from build123d import *

# Parameters (mm, degrees)
BOX_W              = 13.4
BOX_H              = 13.4
BOX_DEPTH          = 14
SKETCH001_R        = 20
POCKET_DEPTH       = 6
POLARPATTERN_COUNT = 5


with BuildPart() as cube:
    # Box → Box (new body)
    with BuildSketch(Plane(origin=(-6.7, -6.7, 10), x_dir=(1, 0, 0), z_dir=(0, 0, 1))):
        with Locations((6.7, 6.7)):
            Rectangle(BOX_W, BOX_H)
    extrude(amount=BOX_DEPTH)


with BuildPart() as body:
    # Sketch → Revolve (revolve)
    with BuildSketch(Plane.XZ):
        with BuildLine():
            Line((78.70723, 18.37), (90, 18.37))
            Line((90, 18.37), (82.032315, 21.27))
            Line((82.032315, 21.27), (82.032315, 23.77))
            Line((82.032315, 23.77), (90, 26.67))
            Line((90, 26.67), (4.86, 26.67))
            Line((4.86, 26.67), (4.86, 10.010664))
            Line((4.86, 10.010664), (11.05, 10.010664))
            Line((11.05, 10.010664), (11.05, 18.37))
            add(Edge.make_bspline(
                [(78.70723, 18.37), (58.452015, 25.146616), (31.574902, 25.049244), (11.05, 18.37)],
                knots=[0, 0, 0, 0, 1, 1, 1, 1], degree=3))
        make_face()
    revolve(axis=Axis((0, 0, 0), (0, 0, 1)))

    # Cut: cut Cube
    add(cube.part, mode=Mode.SUBTRACT)

    # Sketch001 (on Face12 of BaseFeature) → Pocket (cut)
    with BuildSketch(Plane.XY.offset(26.67)):
        with Locations((-32.618477, 27.97224)):
            Circle(SKETCH001_R)
    pocket = extrude(amount=-POCKET_DEPTH, mode=Mode.SUBTRACT)

    # PolarPattern: Pocket ×5 about axis
    polarpattern_axis = Axis((0, 0, 26.67), (0, 0, 1))
    for i in range(1, POLARPATTERN_COUNT):
        add(pocket.rotate(polarpattern_axis, i * 360 / POLARPATTERN_COUNT), mode=Mode.SUBTRACT)


solid = body.part
The listing builds one solid part. Answer for the finished solid, in the listing's coordinates (mm). A direction names the side the tool comes from. Round coordinates to 2 decimals unless told otherwise and drop trailing zeros. Order: outer loops, then holes, each group sorted by start corner. A loop starts at its lowest first (then second) coordinate and runs counter-clockwise, first axis right, second up. Notation, with made-up numbers: (10, -16.75) -> (66, -16.75) arc R20 cw to (66, 22.25) -> close; hole circle Ø1 at (33.25, -37.75). An arc over 180 degrees is marked (long way). Put each result on its own line as item: value.
Q1. Determine the mould class of faces 4 (the cylindrical face through (14.947, 19.728, 24.654)), 5 (the flat face through (19, 1, 26.67)), 6 (the conical face through (38.03, -73.12, 21.13)) for opening direction Y: pulls with the +Y half, pulls with the -Y half, needs draft (parallel to the pull), parting line crosses it, or undercut.
Results list:
face 4: undercut
face 5: needs draft
face 6: parting line crosses it
Q2. Which of the six approach directions +Z, -Z, +X, -X, +Y, -Y give full straight-line access (tool end or side, diameter ignored) to faces 1 (the cylindrical face through (-0.5, -24.75, 24.65)), 2 (the conical face through (-82.45, 3.63, 23.95)), 3 (the flat face through (0, 6.7, 17))?
Results list:
face 1: +Z, -Z
face 2: none
face 3: -Z
Q3. Section B-B, the plane x = 0 is taken. Count the separate pieces of the cut face and the enclosed holes in it, and give its area (3 significant figures).
Results list:
separate pieces: 4
enclosed holes: 0
area: 707 mm^2
Q4. Each of these flat-tipped pins is pushed along its axis until it touches: P1, Ø6, axis at y = 5, z = 20, coming from the -X side; P2, Ø1.5, axis at x = 68, y = -9.5, coming from the -Z side; P3, Ø10, axis at x = 52, y = 65.5, coming from the -Z side. Where does it stop, or does it pass through?
Results list:
P1: x = -89.97
P2: z = 20.91
P3: z = 18.37
Q5. Consider line 1 along Z through (x, y) = (36.5, -70); line 2 along Z through (x, y) = (36, 79.5); line 3 along X through (y, z) = (-67, 21.5). Determine where each line is inside the solid, lowest interval first.
Results list:
line 1: 18.37 to 26.67
line 2: 18.37 to 19.36, 25.68 to 26.67
line 3: -47.33 to 47.33
Q6. Section A-A, the plane z = 12.5 is taken. Write down the section's boundary in (x, y).
Results list:
outline: circle Ø22.1 at (0, 0); hole (-6.7, -6.7) -> (6.7, -6.7) -> (6.7, 6.7) -> (-6.7, 6.7) -> close
